from build123d import *

# Parameters (mm, degrees)
F0_W           = 350
F0_H           = 65
F1_DEPTH       = 30
F3_D           = 11
F3_CBORE_D     = 18
F3_CBORE_DEPTH = 10
F4_SIZE2       = 34.6410161514
F4_SIZE        = 20
F4_2_SIZE2     = 34.6410161514
F4_2_SIZE      = 20


with BuildPart() as f1:
    # F0 (on Top) → F1 (new body)
    with BuildSketch(Plane.XY):
        Rectangle(F0_W, F0_H)
    extrude(amount=F1_DEPTH)

    # F3 (through all)
    with Locations(Plane.XY.offset(30)):
        with Locations((-48, 15), (48, 15), (48, -15), (-48, -15)):
            CounterBoreHole(F3_D / 2, F3_CBORE_D / 2, F3_CBORE_DEPTH)

    # F4
    f4_edges = [f1.edges().sort_by_distance(p)[0] for p in [
        (-175, 0, 30),
    ]]
    f4_side = f1.faces().sort_by_distance((-175, 0, 15))[0]
    chamfer(f4_edges, length=F4_SIZE, length2=F4_SIZE2, reference=f4_side)

    # F4#2
    f4_2_edges = [f1.edges().sort_by_distance(p)[0] for p in [
        (175, 0, 30),
    ]]
    f4_2_side = f1.faces().sort_by_distance((175, 0, 15))[0]
    chamfer(f4_2_edges, length=F4_2_SIZE, length2=F4_2_SIZE2, reference=f4_2_side)


solid = f1.part
The listing builds one solid part. Answer for the finished solid, in the listing's coordinates (mm). A direction names the side the tool comes from. Round coordinates to 2 decimals unless told otherwise and drop trailing zeros. Order: outer loops, then holes, each group sorted by start corner. A loop starts at its lowest first (then second) coordinate and runs counter-clockwise, first axis right, second up. Notation, with made-up numbers: (33, 41.25) -> (89, 41.25) arc R14 ccw to (89, 56.25) -> close; hole circle Ø3 at (44.25, 66.5). An arc over 180 degrees is marked (long way). Write each question's results on one line, items separated by ' | '. Start each with the question number.
Q1. Which of the six approach directions +Z, -Z, +X, -X, +Y, -Y give full straight-line access (tool end or side, diameter ignored) to faces 1 (the flat face through (-2, -32.5, 15)), 2 (the cylindrical face through (40.86, -20.48, 25.07))?
Q2. Find section C-C (z = 23.5). Determine the outline of the cut face in (x, y), then the cut area to 3 significant figures.
Q3. Each of these flat-tipped pins is pushed along its axis until it touches: pin 1 (14.5 mm diameter, centred on x = -52.5, y = 11.5, fed in from +Z); pin 2 (8 mm diameter, centred on y = 0, z = 16.5, fed in from -X); pin 3 (5.5 mm diameter, centred on x = -46.5, y = -19, fed in from +Z); pin 4 (10 mm diameter, centred on x = 48, y = 15, fed in from -Z). Where does it stop, or does it pass through?
Q4. Find section A-A (x = -48). Determine the outline of the cut face in (y, z).
Q5. Find section B-B (y = -15). Determine the outline of the cut face in (x, z), then the cut area to 3 significant figures.
Q6. Find section D-D (y = 28.5). Determine the outline of the cut face in (x, z), then the cut area to 3 significant figures.
Q7. The mould has two halves that part along X. Classify faces 3 (the flat face through (-2, 32.5, 15)), 4 (the flat face through (52, 19, 20)), 5 (the flat face through (-157.44, -0.45, 20.14)): pulls with the +X half, pulls with the -X half, needs draft (parallel to the pull), parting line crosses it, or undercut.
Q8. Straight lines are drawn through the part: probe 1 along Y at (x, z) = (-48, 27); probe 2 along Y at (x, z) = (48, 11); probe 3 along X at (y, z) = (-14, 7.5). For each, find the intervals that lie inside material, in ascending order. Write a range as from..to.
Worked answers:
1) face 1: +Z, -Z, +X, -X, -Y | face 2: +Z
2) outline: (-151.62, -32.5) -> (151.62, -32.5) -> (151.62, 32.5) -> (-151.62, 32.5) -> close; hole circle Ø18 at (-48, -15); hole circle Ø18 at (-48, 15); hole circle Ø18 at (48, -15); hole circle Ø18 at (48, 15) | area: 18,700 mm2
3) pin 1: stops at z = 30 | pin 2: stops at x = -170.67 | pin 3: stops at z = 20 | pin 4: passes through
4) outline: (-32.5, 0) -> (-20.5, 0) -> (-20.5, 20) -> (-24, 20) -> (-24, 30) -> (-32.5, 30) -> close; (-9.5, 0) -> (9.5, 0) -> (9.5, 20) -> (6, 20) -> (6, 30) -> (-6, 30) -> (-6, 20) -> (-9.5, 20) -> close; (20.5, 0) -> (32.5, 0) -> (32.5, 30) -> (24, 30) -> (24, 20) -> (20.5, 20) -> close
5) outline: (-175, 0) -> (-53.5, 0) -> (-53.5, 20) -> (-57, 20) -> (-57, 30) -> (-140.36, 30) -> (-175, 10) -> close; (-42.5, 0) -> (42.5, 0) -> (42.5, 20) -> (39, 20) -> (39, 30) -> (-39, 30) -> (-39, 20) -> (-42.5, 20) -> close; (53.5, 0) -> (175, 0) -> (175, 10) -> (140.36, 30) -> (57, 30) -> (57, 20) -> (53.5, 20) -> close | area: 9,010 mm2
6) outline: (-175, 0) -> (175, 0) -> (175, 10) -> (140.36, 30) -> (-140.36, 30) -> (-175, 10) -> close | area: 9,810 mm2
7) face 3: needs draft | face 4: undercut | face 5: pulls with the -X half
8) probe 1: y = -32.5..-24, -6..6, 24..32.5 | probe 2: y = -32.5..-20.5, -9.5..9.5, 20.5..32.5 | probe 3: x = -175..-53.41, -42.59..42.59, 53.41..175
